For this review, use the dimensioned drawing (mm, ordinates from the lowest corner) and the shaded views. A direction names the side the tool comes from. Coordinates: 2 decimals unless noted, no trailing zeros. Loops run counter-clockwise (first coordinate to the right, second up) from the corner with the lowest first, then second, coordinate; pieces in that order, holes last.
1. Machinability: for the marked faces 1, 2, 3, 4 and 5, which of the approach directions +Z, -Z, +X, -X, +Y, -Y give a long, thin tool a straight path to every point of the face, cutting with its end or side? Answer none if there is none.
2. Take a section at D-D, the plane y = 36.5. State the section outline as (x, z) points.
3. Take a section at A-A, the plane x = 27.5. State the section outline as (y, z) points, then the cut area to 3 significant figures.
4. Take a section at C-C, the plane z = 14.5. State the section outline as (x, y) points.
5. Mouldability with a two-part tool opening along Y and no side actions: class the marked faces 6, 7 and 8 as pulls with the +Y half, pulls with the -Y half, needs draft (parallel to the pull), parting line crosses it, or undercut.
6. Clearance check with flat-ended pins moving along their axes: P1, Ø5, axis at y = 30.5, z = 14.5, coming from the -X side; P2, Ø4.5, axis at x = 47.5, y = 11.5, coming from the +Z side; P3, Ø12, axis at x = 6, z = 15.5, coming from the +Y side. State where each tip first meets the part, or that it passes through.
7. To check wall thickness, follow probe 1 along Y at (x, z) = (27.5, 1.35); probe 2 along Y at (x, z) = (19.5, 11); probe 3 along X at (y, z) = (28, 9.75). State the ranges of each line that lie inside material, in increasing order.
8. Take a section at B-B, the plane y = 11.5. State the section outline as (x, z) points, then the cut area to 3 significant figures.
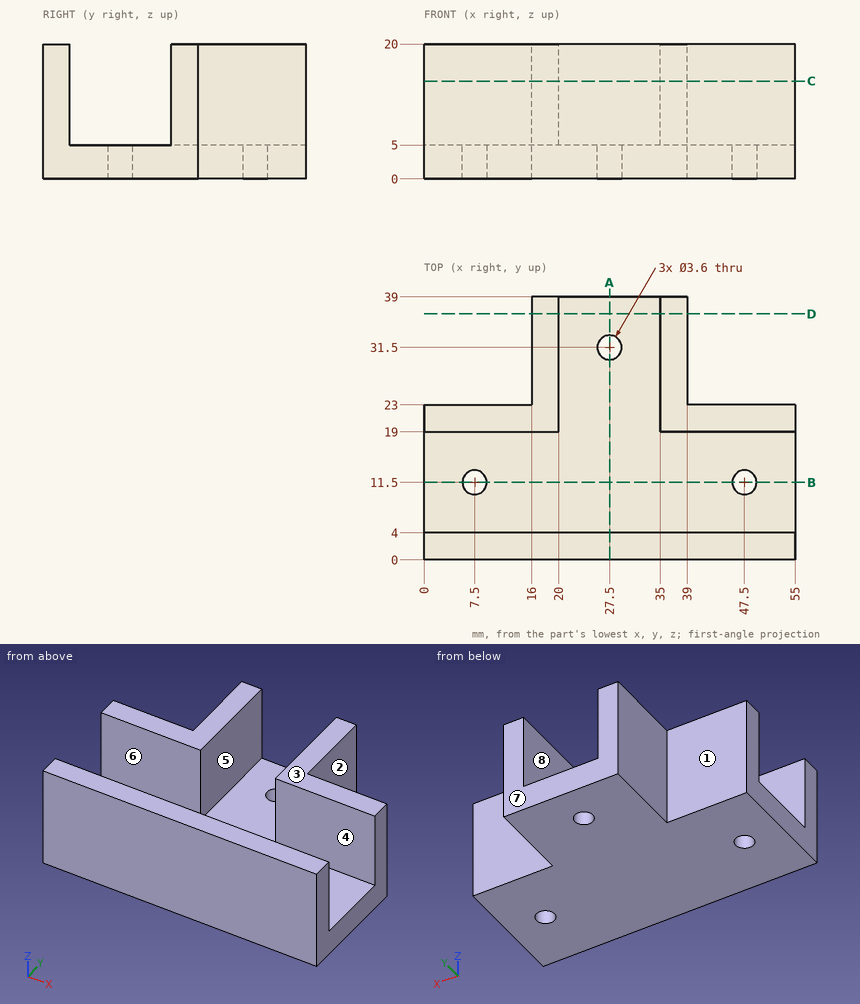
Results list:
1. face 1: +Z, -Z, -X, +Y
1. face 2: +Z, -Z, +X, +Y
1. face 3: +Z, +X, -X, +Y, -Y
1. face 4: +Z, +X, -X
1. face 5: +Z, +Y
2. outline: (16, 0) - (39, 0) - (39, 20) - (35, 20) - (35, 5) - (20, 5) - (20, 20) - (16, 20) - close
3. outline: (0, 0) - (29.7, 0) - (29.7, 5) - (4, 5) - (4, 20) - (0, 20) - close; (33.3, 0) - (39, 0) - (39, 5) - (33.3, 5) - close
3. area: 237 mm2
4. outline: (0, 0) - (55, 0) - (55, 4) - (0, 4) - close; (0, 19) - (20, 19) - (20, 39) - (16, 39) - (16, 23) - (0, 23) - close; (35, 19) - (55, 19) - (55, 23) - (39, 23) - (39, 39) - (35, 39) - close
5. face 6: undercut
5. face 7: pulls with the +Y half
5. face 8: needs draft
6. P1: stops at x = 16
6. P2: stops at z = 5
6. P3: stops at y = 23
7. probe 1: y = 0 to 29.7, 33.3 to 39
7. probe 2: y = 0 to 4, 19 to 39
7. probe 3: x = 16 to 20, 35 to 39
8. outline: (0, 0) - (5.7, 0) - (5.7, 5) - (0, 5) - close; (9.3, 0) - (45.7, 0) - (45.7, 5) - (9.3, 5) - close; (49.3, 0) - (55, 0) - (55, 5) - (49.3, 5) - close
8. area: 239 mm2
